```python
from build123d import *

# Parameters (mm, degrees)
F1_DEPTH = 5


with BuildPart() as f1:
    # F0 (on Front) → F1 (new body)
    with BuildSketch(Plane.XZ):
        with BuildLine():
            Line((-21.807785, -1.172308), (-24.221647, -1.172308))
            ThreePointArc((-24.221647, -1.172308), (-14.764985, -19.236884), (5.130451, -23.701075))
            Line((5.130451, -23.701075), (5.130451, -22.882067))
            Line((5.130451, -22.882067), (3.264538, -22.882067))
            Line((3.264538, -22.882067), (3.264538, -20.541335))
            Line((3.264538, -20.541335), (8.456405, -20.541335))
            Line((8.456405, -20.541335), (8.456405, -18.974984))
            Line((8.456405, -18.974984), (10.286748, -18.974984))
            Line((10.286748, -18.974984), (10.286748, -17.197439))
            Line((10.286748, -17.197439), (15.44636, -17.197439))
            Line((15.44636, -17.197439), (15.44636, -15.602398))
            Line((15.44636, -15.602398), (17.285462, -15.602398))
            Line((17.285462, -15.602398), (17.285462, -14.024785))
            Line((17.285462, -14.024785), (13.642496, -14.024785))
            Line((13.642496, -14.024785), (13.642496, -12.465751))
            Line((13.642496, -12.465751), (8.446803, -12.465751))
            Line((8.446803, -12.465751), (8.446803, -10.388738))
            Line((8.446803, -10.388738), (12.081455, -10.388738))
            Line((12.081455, -10.388738), (12.081455, -8.669803))
            Line((12.081455, -8.669803), (12.081455, -8.58615))
            Line((12.081455, -8.58615), (12.14105, -8.58615))
            Line((12.14105, -8.58615), (18.825023, -8.58615))
            Line((18.825023, -8.58615), (18.825023, -7.2836))
            Line((18.825023, -7.2836), (15.464293, -7.2836))
            Line((15.464293, -7.2836), (15.464293, -5.200631))
            Line((15.464293, -5.200631), (23.685775, -5.200631))
            ThreePointArc((23.685775, -5.200631), (24.038243, -3.197714), (24.221647, -1.172308))
            Line((24.221647, -1.172308), (21.807785, -1.172308))
            ThreePointArc((21.807785, -1.172308), (21.838886, -0.129742), (21.820174, 0.913119))
            Line((21.820174, 0.913119), (24.232802, 0.913119))
            ThreePointArc((24.232802, 0.913119), (24.070018, 2.949024), (23.736493, 4.96401))
            Line((23.736493, 4.96401), (13.632283, 4.96401))
            Line((13.632283, 4.96401), (13.632283, 6.956257))
            Line((13.632283, 6.956257), (17.293811, 6.956257))
            Line((17.293811, 6.956257), (17.293811, 8.313401))
            Line((17.293811, 8.313401), (10.260658, 8.313401))
            Line((10.260658, 8.313401), (10.260658, 10.381422))
            Line((10.260658, 10.381422), (15.457919, 10.381422))
            Line((15.457919, 10.381422), (15.457919, 11.972982))
            Line((15.457919, 11.972982), (13.678564, 11.972982))
            Line((13.678564, 11.972982), (13.678564, 13.525478))
            Line((13.678564, 13.525478), (10.285563, 13.525478))
            Line((10.285563, 13.525478), (10.285563, 15.58539))
            Line((10.285563, 15.58539), (11.87324, 15.58539))
            Line((11.87324, 15.58539), (11.87324, 17.176317))
            Line((11.87324, 17.176317), (8.44818, 17.176317))
            Line((8.44818, 17.176317), (8.44818, 19.14476))
            Line((8.44818, 19.14476), (10.285563, 19.14476))
            Line((10.285563, 19.14476), (10.285563, 21.96064))
            ThreePointArc((10.285563, 21.96064), (-12.624615, 20.704627), (-24.232802, 0.913119))
            Line((-24.232802, 0.913119), (-21.820174, 0.913119))
            ThreePointArc((-21.820174, 0.913119), (-21.838886, -0.129742), (-21.807785, -1.172308))
        make_face()
        with BuildLine():
            ThreePointArc((-14.82406, -1.172308), (-14.869774, -0.129914), (-14.84228, 0.913119))
            Line((-14.84228, 0.913119), (14.84228, 0.913119))
            ThreePointArc((14.84228, 0.913119), (14.869774, -0.129914), (14.82406, -1.172308))
            Line((14.82406, -1.172308), (-14.82406, -1.172308))
        make_face(mode=Mode.SUBTRACT)
        with BuildLine():
            ThreePointArc((-11.885257, 18.321967), (-4.965121, 18.18768), (-1.543241, 12.171281))
            ThreePointArc((-1.543241, 12.171281), (-11.41194, 5.786098), (-13.191973, 17.404759))
            ThreePointArc((-13.191973, 17.404759), (-12.564849, 17.900738), (-11.885257, 18.321967))
        make_face(mode=Mode.SUBTRACT)
        with BuildLine():
            Line((12.081455, -8.58615), (12.081455, -8.669803))
            ThreePointArc((12.081455, -8.669803), (12.111325, -8.628028), (12.14105, -8.58615))
            Line((12.14105, -8.58615), (12.081455, -8.58615))
        make_face()
    extrude(amount=F1_DEPTH)


solid = f1.part
```
Geometry check sheet. Reference: the model listing, model coordinates, mm. A direction names the side the tool comes from. Coordinates: 2 decimals unless noted, no trailing zeros. Order: outer loops, then holes, each group sorted by start corner. A loop starts at its lowest first (then second) coordinate and runs counter-clockwise, first axis right, second up.
Q1. Sectioned sample at B-B on z = -0.5. Record the cut outline in (x, y), and give its area (3 significant figures).
Reply:
outline: (-21.83, -5) - (-14.86, -5) - (-14.86, 0) - (-21.83, 0) - close; (14.86, -5) - (21.83, -5) - (21.83, 0) - (14.86, 0) - close
area: 69.7 mm2
Q2. Thickness scan on probe 1 along Z at (x, y) = (10.5, -2.75); probe 2 along Z at (x, y) = (-0.5, -3.3); probe 3 along Z at (x, y) = (-9.5, -2.25). Record the ranges inside material, lowest first.
Reply:
probe 1: z = -17.2 to -12.47, -10.39 to -1.17, 0.91 to 8.31, 10.38 to 13.53, 15.59 to 17.18
probe 2: z = -24.24 to -1.17, 0.91 to 24.24
probe 3: z = -22.31 to -1.17, 0.91 to 5.24, 19.11 to 22.31
Q3. Tool access check on faces 4 (the face through (13.679, -2, 13)), 5 (the face through (13.632, -2, 6)), 6 (the face through (-14.87, -2.46, -0.14)), 7 (the face through (18.825, -2, -8)), 8 (the face through (-23, -2, -1.172)). Record the directions out of +Z, -Z, +X, -X, +Y, -Y that give a thin tool (end or side, any length) a straight path to the whole face; none if there is none.
Reply:
face 4: +Z, +X, +Y, -Y
face 5: +X, +Y, -Y
face 6: +Y, -Y
face 7: -Z, +X, +Y, -Y
face 8: -X, +Y, -Y
Q4. Draft check along Z on faces 1 (the face through (15.458, -2, 11)), 2 (the face through (13, -2, -17.197)), 3 (the face through (15, -2, -8.586)). Enter one of: released by +Z, released by -Z, zero draft, split by the parting line, or undercut.
Reply:
face 1: zero draft
face 2: released by -Z
face 3: undercut
Q5. Sectioned sample at C-C on x = -9.5. Record the cut outline in (y, z).
Reply:
outline: (-5, -22.31) - (0, -22.31) - (0, -1.17) - (-5, -1.17) - close; (-5, 0.91) - (0, 0.91) - (0, 5.24) - (-5, 5.24) - close; (-5, 19.11) - (0, 19.11) - (0, 22.31) - (-5, 22.31) - close
Q6. Sectioned sample at A-A on x = 0. Record the cut outline in (y, z), and give its area (3 significant figures).
Reply:
outline: (-5, -24.25) - (0, -24.25) - (0, -1.17) - (-5, -1.17) - close; (-5, 0.91) - (0, 0.91) - (0, 24.25) - (-5, 24.25) - close
area: 232 mm2
Q7. Depth check by flat-ended pin: pin 1 Ø1.5 at (x, y) = (-5, -2) entering from -Z; pin 2 Ø1.5 at (x, y) = (12.5, -3) entering from -Z; pin 3 Ø2.5 at (y, z) = (-2.5, -22) entering from +X; pin 4 Ø8.5 at (x, z) = (-8.54, 12.17) entering from +Y. Enter the tip coordinate at first touch or a pass-through.
Reply:
pin 1: stops at z = -23.87
pin 2: stops at z = -17.2
pin 3: stops at x = 5.13
pin 4: passes through
Q8. Sectioned sample at D-D on y = -2.05. Give the number of separate pieces and of enclosed holes in the cut face, and give its area (3 significant figures).
Reply:
separate pieces: 1
enclosed holes: 2
area: 1,380 mm2
